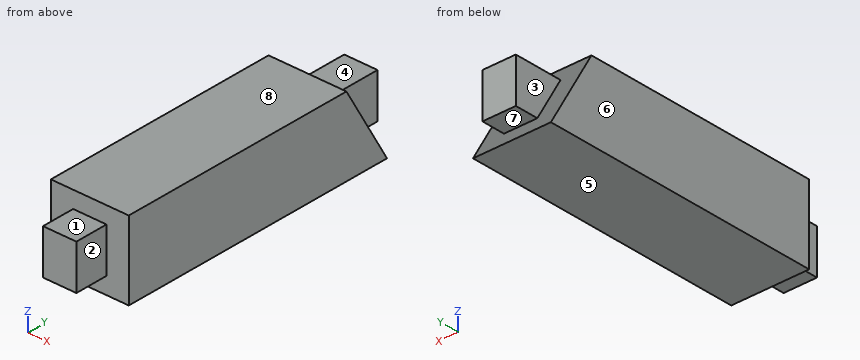
from build123d import *

# Parameters (mm, degrees)
F0_W     = 381
F0_H     = 88.9
F1_DEPTH = 44.45
F4_W     = 88.9
F4_H     = 88.9
F4_W_2   = 38.1
F4_H_2   = 50.8
F5_REACH = 193.287585695
F6_W     = 88.9
F6_H     = 88.9
F6_W_2   = 38.1
F6_H_2   = 50.8
F7_DEPTH = 38.1


with BuildPart() as f1:
    # F0 (on Right) → F1 (new body, symmetric)
    with BuildSketch(Plane.YZ):
        Rectangle(F0_W, F0_H)
    extrude(amount=F1_DEPTH, both=True)

    f5_end = Plane(origin=(0, 111.4494145991, 64.3453495198), x_dir=(0, -0.5, 0.8660254038), z_dir=(0, 0.8660254038, 0.5))
    # F4 (on face) → F5 (cut, up to a plane its end follows)
    with BuildSketch(Plane(origin=(0, 190.5, 0), x_dir=(-1, 0, 0), z_dir=(0, 1, 0))):
        Rectangle(F4_W, F4_H)
        Rectangle(F4_W_2, F4_H_2, mode=Mode.SUBTRACT)
    f5_long = extrude(amount=-F5_REACH, mode=Mode.PRIVATE)
    add(split(f5_long, bisect_by=f5_end, keep=Keep.TOP, mode=Mode.PRIVATE), mode=Mode.SUBTRACT)

    # F6 (on face) → F7 (cut)
    with BuildSketch(Plane.XZ.offset(190.5)):
        Rectangle(F6_W, F6_H)
        Rectangle(F6_W_2, F6_H_2, mode=Mode.SUBTRACT)
    extrude(amount=-F7_DEPTH, mode=Mode.SUBTRACT)


solid = f1.part
Read the model definition and answer for the solid it produces. Units are mm, in the model's axes. Face numbers are marked on the shaded views. A direction names the side the tool comes from. Coordinates: 2 decimals unless noted, no trailing zeros. Loops run counter-clockwise (first coordinate to the right, second up) from the corner with the lowest first, then second, coordinate; pieces in that order, holes last.
Q1. The part is cut by section D-D on x = 25. Write down the section's boundary in (y, z), and give its area (3 significant figures).
Q2. The part is cut by section A-A on x = -7. Write down the section's boundary in (y, z), and give its area (3 significant figures).
Q3. The mould has two halves that part along Z. Classify the marked faces 5, 6, 7 and 8: +Z half, -Z half, draft (parallel to the pull), parting line (faces both ways), or undercut.
Q4. Consider probe 1 along X at (y, z) = (-167, 0.5); probe 2 along Z at (x, y) = (15, 144.5); probe 3 along Z at (x, y) = (-17.5, 174.5). Determine where each line is inside the solid, lowest interval first.
Q5. The part is cut by section C-C on y = 139.5. Write down the section's boundary in (x, z), and give its area (3 significant figures).
Q6. Each of these flat-tipped pins is pushed along its axis until it touches: pin 1 Ø3 at (x, z) = (35.5, -7.5) entering from -Y; pin 2 Ø6 at (x, z) = (-29, -35) entering from +Y; pin 3 Ø4 at (x, z) = (-33, -14.5) entering from +Y. Where does it stop, or does it pass through?
Q7. Which of the six approach directions +Z, -Z, +X, -X, +Y, -Y give full straight-line access (tool end or side, diameter ignored) to the marked faces 1, 2, 3 and 4?
Q8. The part is cut by section B-B on z = 17.5. Write down the section's boundary in (x, y).
Results below:
1. outline: (-152.4, -44.45) - (174.26, -44.45) - (122.94, 44.45) - (-152.4, 44.45) - close
1. area: 26,800 mm2
2. outline: (-190.5, -25.4) - (-152.4, -25.4) - (-152.4, -44.45) - (174.26, -44.45) - (163.26, -25.4) - (190.5, -25.4) - (190.5, 25.4) - (133.93, 25.4) - (122.94, 44.45) - (-152.4, 44.45) - (-152.4, 25.4) - (-190.5, 25.4) - close
2. area: 30,800 mm2
3. face 5: -Z half
3. face 6: draft
3. face 7: undercut
3. face 8: +Z half
4. probe 1: x = -19.05 to 19.05
4. probe 2: z = -44.45 to 25.4
4. probe 3: z = -25.4 to 25.4
5. outline: (-44.45, -44.45) - (44.45, -44.45) - (44.45, 15.76) - (19.05, 15.76) - (19.05, 25.4) - (-19.05, 25.4) - (-19.05, 15.76) - (-44.45, 15.76) - close
5. area: 5,720 mm2
6. pin 1: stops at y = -152.4
6. pin 2: stops at y = 170.54
6. pin 3: stops at y = 158.13
7. face 1: +Z, +X, -X, -Y
7. face 2: +Z, -Z, +X, -Y
7. face 3: +Z, -X, +Y
7. face 4: +Z, +X, -X, +Y
8. outline: (-44.45, -152.4) - (-19.05, -152.4) - (-19.05, -190.5) - (19.05, -190.5) - (19.05, -152.4) - (44.45, -152.4) - (44.45, 138.5) - (19.05, 138.5) - (19.05, 190.5) - (-19.05, 190.5) - (-19.05, 138.5) - (-44.45, 138.5) - close
